The listing builds one solid part. Answer for the finished solid, in the listing's coordinates (mm). Face numbers are marked on the shaded views. A direction names the side the tool comes from. Round coordinates to 2 decimals unless told otherwise and drop trailing zeros. Write each loop counter-clockwise with the first axis right and the second up, starting at its lowest first coordinate (ties: lowest second). Pieces come first, ordered by that corner, then holes. Notation, with made-up numbers: M 43,31 L 79,31 A19 ccw 79,48 Z; hole C -10.5,31 d7. An arc over 180 degrees is marked long. One line per item, written item: value. Start each with the question number.
(1) Section B-B (x = 18) is taken. Determine the outline of the cut face in (y, z).
(2) Section A-A (y = 7.5) is taken. Determine the outline of the cut face in (x, z).
(3) Consider probe 1 along Z at (x, y) = (22.5, -13.5); probe 2 along X at (y, z) = (12, 10.25); probe 3 along X at (y, z) = (-7, 5). Determine where each line is inside the solid, lowest interval first.
(4) For a pull along X with two mould halves and no side action, classify the marked faces 3, 4 and 5 as released by +X, released by -X, zero draft, split by the parting line, or undercut.
(5) For the marked faces 1 and 2, determine the directions among +Z, -Z, +X, -X, +Y, -Y from which every point of the face is accessible in a straight line to the end or side of a thin tool.
(6) Section C-C (z = 4.75) is taken. Determine the outline of the cut face in (x, y), plus the area to 3 significant figures.
(7) Given P1, Ø4, axis at y = 0, z = 3, coming from the -X side; P2, Ø1, axis at x = -15, z = 5, coming from the +Y side; P3, Ø2, axis at x = -8, z = 2.5, coming from the +Y side; P4, Ø6, axis at x = -9.5, z = 11, coming from the -Y side, each flat-ended and moving along its own axis, determine where each tip first touches the part or whether it passes through.
(8) Section D-D (z = 1) is taken. Determine the outline of the cut face in (x, y), plus the area to 3 significant figures.
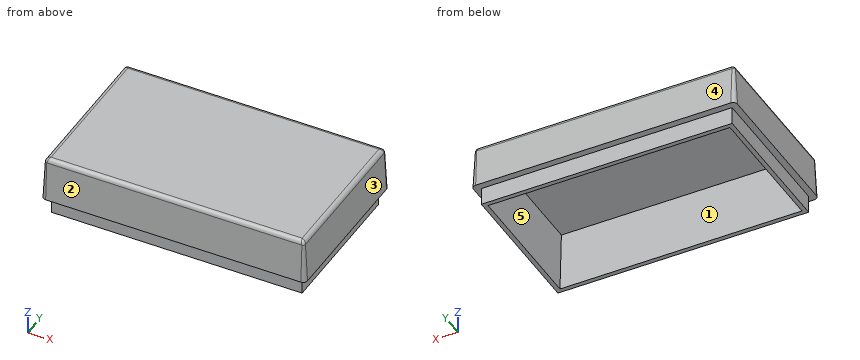
Autodesk Inventor part; units mm, degrees
ref_plane "YZ Plane" through (0, 0, 0) normal (1, 0, 0) x (0, 1, 0)
ref_plane "XZ Plane" through (0, 0, 0) normal (0, 1, 0) x (-1, 0, 0)
ref_plane "XY Plane" through (0, 0, 0) normal (0, 0, 1) x (1, 0, 0)
sketch "Эскиз1" plane through (0, 0, 0) normal (0, 0, 1) x (1, 0, 0)
  line L0 (-29, 18) -> (29, 18)
  line L1 (30, 17) -> (30, -17)
  line L2 (29, -18) -> (-29, -18)
  line L3 (-30, -17) -> (-30, 17)
  arc A0 (-29, 18) -> (-30, 17) centre (-29, 17) ccw
  arc A1 (-30, -17) -> (-29, -18) centre (-29, -17) ccw
  arc A2 (29, -18) -> (30, -17) centre (29, -17) ccw
  arc A3 (30, 17) -> (29, 18) centre (29, 17) ccw
  point P0 (0, 0)
  point P1 (-30, 18)
  point P2 (30, 18)
  point P3 (-30, -18)
  dimension "d0" = 60
  dimension "d1" = 36
  dimension "d2" = 18
  dimension "d3" = 30
  dimension "d4" = 1
extrude "Выдавливание1" add sketch "Эскиз1" along normal blind 4
sketch "Эскиз3" plane through (0, 0, 4) normal (0, 0, 1) x (1, 0, 0)
  line L0 (-29, 18) -> (29, 18)
  line L1 (30, 17) -> (30, -17)
  line L2 (29, -18) -> (-29, -18)
  line L3 (-30, -17) -> (-30, 17)
  line L4 (30, -17) -> (30, 17)
  line L5 (-29, -18) -> (29, -18)
  line L6 (-30, 17) -> (-30, -17)
  line L7 (29, 18) -> (-29, 18)
  arc A0 (-29, 18) -> (-30, 17) centre (-29, 17) ccw
  arc A1 (-30, -17) -> (-29, -18) centre (-29, -17) ccw
  arc A2 (29, -18) -> (30, -17) centre (29, -17) ccw
  arc A3 (30, 17) -> (29, 18) centre (29, 17) ccw
  point P0 (0, 0)
  dimension "d7" = 0
  dimension "d8" = 0
  dimension "d9" = 0
  dimension "d10" = 0
  dimension "d11" = 1
extrude "Выдавливание2" add sketch "Эскиз3" along normal blind 10 draft -3
sketch "Эскиз4" plane through (0, 0, 0) normal (0, 0, -1) x (-1, 0, 0)
  line L0 (-27.5, 15.5) -> (27.5, 15.5)
  line L1 (27.5, 15.5) -> (27.5, -15.5)
  line L2 (27.5, -15.5) -> (-27.5, -15.5)
  line L3 (-27.5, -15.5) -> (-27.5, 15.5)
  point P0 (0, 0)
  dimension "d14" = 15.5
  dimension "d15" = 31
  dimension "d16" = 27.5
  dimension "d17" = 55
extrude "Выдавливание3" cut sketch "Эскиз4" against normal blind 13 draft -3
sketch "Эскиз5" plane through (0, 0, 0) normal (0, 0, -1) x (-1, 0, 0)
  line L0 (-28.5, 16.5) -> (28.5, 16.5)
  line L1 (28.5, 16.5) -> (28.5, -16.5)
  line L2 (28.5, -16.5) -> (-28.5, -16.5)
  line L3 (-28.5, -16.5) -> (-28.5, 16.5)
  line L4 (-29, 18) -> (29, 18)
  line L5 (-30, -17) -> (-30, 17)
  line L6 (29, -18) -> (-29, -18)
  line L7 (30, 17) -> (30, -17)
  line L8 (-29, 18) -> (29, 18)
  line L9 (30, 17) -> (30, -17)
  line L10 (29, -18) -> (-29, -18)
  line L11 (-30, -17) -> (-30, 17)
  arc A0 (-29, 18) -> (-30, 17) centre (-29, 17) ccw
  arc A1 (-30, -17) -> (-29, -18) centre (-29, -17) ccw
  arc A2 (29, -18) -> (30, -17) centre (29, -17) ccw
  arc A3 (30, 17) -> (29, 18) centre (29, 17) ccw
  point P0 (0, 0)
  point P1 (29, 18)
  dimension "d20" = 1.5
  dimension "d21" = 1.5
  dimension "d22" = 1.5
  dimension "d23" = 1.5
  dimension "d24" = 0
  dimension "d25" = 0
  dimension "d26" = 0
  dimension "d27" = 0
  dimension "d28" = 1
extrude "Выдавливание4" cut sketch "Эскиз5" against normal blind 4
fillet "Сопряжение1" radius 1 8 edges at (-29.3365, -17.3365, 14) (-29.4759, 0, 14) (-29.3365, 17.3365, 14) (0, 17.4759, 14) (29.3365, 17.3365, 14) (29.4759, 0, 14) (29.3365, -17.3365, 14) (0, -17.4759, 14)
properties part number "case_up" material "Пластик АБС"
Recorded:
1. outline: M -18,4 L -16.5,4 L -16.5,0 L -15.5,0 L -14.82,13 L 14.82,13 L 15.5,0 L 16.5,0 L 16.5,4 L 18,4 L 17.53,13.05 A1 ccw 16.53,14 L -16.53,14 A1 ccw -17.53,13.05 Z
2. outline: M -30,4 L -28.5,4 L -28.5,0 L -27.5,0 L -26.82,13 L 26.82,13 L 27.5,0 L 28.5,0 L 28.5,4 L 30,4 L 29.53,13.05 A1 ccw 28.53,14 L -28.53,14 A1 ccw -29.53,13.05 Z
3. probe 1: z = 13 to 14
3. probe 2: x = -29.67 to -26.96, 26.96 to 29.67
3. probe 3: x = -29.95 to -27.24, 27.24 to 29.95
4. face 3: released by +X
4. face 4: zero draft
4. face 5: undercut
5. face 1: -Z
5. face 2: +Z, +X, -X, -Y
6. outline: M -29.96,-17 A0.96 ccw -29,-17.96 L 29,-17.96 A0.96 ccw 29.96,-17 L 29.96,17 A0.96 ccw 29,17.96 L -29,17.96 A0.96 ccw -29.96,17 Z; hole M -27.25,-15.25 L 27.25,-15.25 L 27.25,15.25 L -27.25,15.25 Z
6. area: 489 mm2
7. P1: stops at x = -30
7. P2: stops at y = 17.97
7. P3: stops at y = 16.5
7. P4: stops at y = -17.79
8. outline: M -28.5,-16.5 L 28.5,-16.5 L 28.5,16.5 L -28.5,16.5 Z; hole M -27.45,-15.45 L 27.45,-15.45 L 27.45,15.45 L -27.45,15.45 Z
8. area: 185 mm2
